The model under review builds one solid part; all positions refer to its coordinate system, in mm. A direction names the side the tool comes from. Round coordinates to 2 decimals unless told otherwise and drop trailing zeros. Loops run counter-clockwise (first coordinate to the right, second up) from the corner with the lowest first, then second, coordinate; pieces in that order, holes last. Notation, with made-up numbers: (-16, 26.5) - (13, 26.5) arc R25 ccw to (13, 62.5) - close; hole circle Ø5 at (43.25, 21). An arc over 180 degrees is marked (long way). Answer as CSV lines item,"result".
from build123d import *

# Parameters (mm, degrees)
BOSS_EXTRUDE1_DEPTH     = 14
SKETCH2_R               = 2.6
SKETCH2_R_2             = 2.5
SKETCH2_R_3             = 3
SKETCH2_W               = 275
SKETCH2_H               = 75
CUT_EXTRUDE1_DEPTH      = 1
CUT_EXTRUDE1_DEPTH_BACK = 15
CHAMFER1_SIZE           = 40


with BuildPart() as part:
    # Sketch1 → Boss-Extrude1 (new body)
    with BuildSketch(Plane(origin=(0, 0, 0), x_dir=(1, 0, 0), z_dir=(0, 1, 0))):
        Polygon((-75, -40), (-75, 40), (75, 40), (75, -40), (200, -40), (200, -180), (-200, -180), (-200, -40), align=None)
    extrude(amount=BOSS_EXTRUDE1_DEPTH)

    # Sketch2 → Cut-Extrude1 (cut, two sides)
    with BuildSketch(Plane(origin=(0, 14, 0), x_dir=(1, 0, 0), z_dir=(0, 1, 0))) as cut_extrude1_sk:
        with Locations((-67.5, 25)):
            Circle(SKETCH2_R)
        with Locations((-67.5, 0)):
            Circle(SKETCH2_R)
        with Locations((-182, -168)):
            Circle(SKETCH2_R_2)
        with Locations((-182, -112)):
            Circle(SKETCH2_R_2)
        with Locations((-37.5, 17.5)):
            Circle(SKETCH2_R_3)
        with Locations((-37.5, -87.5)):
            Circle(SKETCH2_R_3)
        with Locations((37.5, -87.5)):
            Circle(SKETCH2_R_3)
        with Locations((37.5, 17.5)):
            Circle(SKETCH2_R_3)
        with Locations((182, -112)):
            Circle(SKETCH2_R_2)
        with Locations((182, -168)):
            Circle(SKETCH2_R_2)
        with Locations((67.5, 0)):
            Circle(SKETCH2_R)
        with Locations((67.5, 25)):
            Circle(SKETCH2_R)
        with Locations((0, -142.5)):
            Rectangle(SKETCH2_W, SKETCH2_H)
    extrude(amount=CUT_EXTRUDE1_DEPTH, mode=Mode.SUBTRACT)
    extrude(cut_extrude1_sk.sketch, amount=-CUT_EXTRUDE1_DEPTH_BACK, mode=Mode.SUBTRACT)

    # Chamfer1
    chamfer1_edges = [part.edges().sort_by_distance(p)[0] for p in [
        (200, 7, 40),
        (-200, 7, 40),
        (-137.5, 7, 105),
        (137.5, 7, 105),
    ]]
    chamfer(chamfer1_edges, length=CHAMFER1_SIZE)


solid = part.part
1. Draft analysis for pull direction X (two halves, no side actions). For faces 6 (the face through (3, 0, 68)), 7 (the face through (-200, 7, 131)), 8 (the face through (-137.5, 7, 163)), state which applies: +X half, -X half, draft (parallel to the pull), parting line (faces both ways), or undercut.
Numbers:
face 6,"draft"
face 7,"-X half"
face 8,"undercut"
2. Take a section at C-C (x = 119). State the section outline as (y, z) points, plus the area to 3 significant figures.
Numbers:
outline,"(0, 40) - (14, 40) - (14, 126.5) - (0, 126.5) - close"
area,"1,210 mm²"
3. Wall thickness on probe 1 along X at (y, z) = (6.75, 0); probe 2 along Z at (x, y) = (37.5, 7.5); probe 3 along X at (y, z) = (3, 149): over which ranges is each line inside the solid? List them lowest first.
Numbers:
probe 1,"x = -75 to -70.1, -64.9 to 64.9, 70.1 to 75"
probe 2,"z = -40 to -20.5, -14.5 to 84.5, 90.5 to 105"
probe 3,"x = -200 to -137.5, 137.5 to 200"
4. Take a section at B-B (y = 3.75). State how many separate pieces and enclosed holes the cut face has, plus the area to 3 significant figures.
Numbers:
separate pieces,"1"
enclosed holes,"12"
area,"47,100 mm²"
5. Tool access review of faces 1 (the face through (-168, 7, 180)), 2 (the face through (200, 7, 129)), 3 (the face through (-1, 7, 105)), 4 (the face through (75, 7, -1)), 5 (the face through (-75, 7, 1)): name each direction out of +Z, -Z, +X, -X, +Y, -Y from which nothing blocks a thin tool from reaching the whole face with its end or side.
Numbers:
face 1,"+Z, +X, -X, +Y, -Y"
face 2,"+Z, -Z, +X, +Y, -Y"
face 3,"+Z, +Y, -Y"
face 4,"-Z, +X, +Y, -Y"
face 5,"-Z, -X, +Y, -Y"
6. Take a section at A-A (z = 141). State the section outline as (x, y) points, plus the area to 3 significant figures.
Numbers:
outline,"(-200, 0) - (-133.5, 0) - (-133.5, 14) - (-200, 14) - close; (133.5, 0) - (200, 0) - (200, 14) - (133.5, 14) - close"
area,"1,860 mm²"
7. Clearance check with flat-ended pins moving along their axes: pin 1 (8.5 mm diameter, centred on x = -67.5, z = -25, fed in from +Y); pin 2 (8 mm diameter, centred on x = 105, y = 8.5, fed in from +Z); pin 3 (8 mm diameter, centred on x = -127.5, y = 9, fed in from -Z); pin 4 (4 mm diameter, centred on x = -15, y = 4, fed in from +Z). State where each tip first meets the part, or that it passes through.
Numbers:
pin 1,"stops at y = 14"
pin 2,"stops at z = 116.5"
pin 3,"stops at z = 40"
pin 4,"stops at z = 105"
8. Take a section at D-D (z = 32). State the section outline as (x, y) points.
Numbers:
outline,"(-75, 0) - (75, 0) - (75, 14) - (-75, 14) - close"
